The model under review builds one solid part; all positions refer to its coordinate system, in mm. Face numbers are marked on the shaded views. A direction names the side the tool comes from. Round coordinates to 2 decimals unless told otherwise and drop trailing zeros. Order: outer loops, then holes, each group sorted by start corner. A loop starts at its lowest first (then second) coordinate and runs counter-clockwise, first axis right, second up. Notation, with made-up numbers: M -1.75,81 L 47.25,81 A25 ccw 47.25,109 Z; hole C 47,4.5 d9. An arc over 180 degrees is marked long. Answer as a JSON object with one key per item and string values. Group by question number.
1) For the marked faces 4 and 5, list the 3-axis set-ups (+Z, -Z, +X, -X, +Y, -Y) from which the entire face can be reached by the end or side of a thin tool; tool diameter is ignored.
2) To check wall thickness, follow line 1 (Y direction, x = 1.5, z = 3.75); line 2 (X direction, y = 85.5, z = 4); line 3 (X direction, y = 93, z = 8). State the ranges of each line that lie inside material, in increasing order.
3) Consider section A-A, the plane x = -28.5. Write out the cut boundary in (y, z).
4) Insertion check: pin 1 Ø8 at (x, y) = (-24.5, 39.5) entering from +Z; pin 2 Ø2.5 at (x, z) = (-26.5, 6) entering from +Y; pin 3 Ø3 at (y, z) = (50, 4.5) entering from -X; pin 4 Ø2.5 at (x, y) = (-29.5, 117) entering from +Z. Each pin has a flat end and moves straight along its axis. Give the tip position at first contact, or say it passes through.
5) Consider section B-B, the plane y = 38. Write out the cut boundary in (x, z).
6) The part is to be moulded in two halves that separate along Y. For the marked faces 1, 2 and 3, say which applies: +Y half, -Y half, draft (parallel to the pull), parting line (faces both ways), or undercut.
```python
from build123d import *

# Parameters (mm, degrees)
F0_W      = 79.5
F0_H      = 118.5
F1_DEPTH  = 10
F3_R      = 7
F5_DEPTH  = 3.5
F6_R      = 0.8
F8_DEPTH  = 3.5
F9_R      = 2
F10_DEPTH = 4.5
F2_W      = 14.5
F2_H      = 4.5
F11_DEPTH = 4
F13_DEPTH = 9
F14_DEPTH = 25
F15_R     = 2


with BuildPart() as f1:
    # F0 (on Top) → F1 (new body)
    with BuildSketch(Plane.XY):
        with Locations((0, 59.25)):
            Rectangle(F0_W, F0_H)
    extrude(amount=F1_DEPTH)

    # F3
    f3_edges = [f1.edges().sort_by_distance(p)[0] for p in [
        (-39.75, 118.5, 5),
        (-39.75, 0, 5),
        (39.75, 0, 5),
        (39.75, 118.5, 5),
    ]]
    fillet(f3_edges, radius=F3_R)

    # F4 (on face) → F5 (cut)
    with BuildSketch(Plane.XY.offset(10)):
        with BuildLine():
            Line((32.75, 116.5), (-32.75, 116.5))
            ThreePointArc((-32.75, 116.5), (-36.2855339059, 115.0355339059), (-37.75, 111.5))
            Line((-37.75, 111.5), (-37.75, 7))
            ThreePointArc((-37.75, 7), (-36.2855339059, 3.4644660941), (-32.75, 2))
            Line((-32.75, 2), (32.75, 2))
            ThreePointArc((32.75, 2), (36.2855339059, 3.4644660941), (37.75, 7))
            Line((37.75, 7), (37.75, 111.5))
            ThreePointArc((37.75, 111.5), (36.2855339059, 115.0355339059), (32.75, 116.5))
        make_face()
    extrude(amount=-F5_DEPTH, mode=Mode.SUBTRACT)

    # F6
    f6_edges = [f1.edges().sort_by_distance(p)[0] for p in [
        (0, 118.5, 0),
        (37.699747, 116.449747, 0),
        (-37.699747, 116.449747, 0),
        (39.75, 59.25, 0),
        (-39.75, 59.25, 0),
        (37.699747, 2.050253, 0),
        (-37.699747, 2.050253, 0),
        (0, 0, 0),
    ]]
    fillet(f6_edges, radius=F6_R)

    # F7 (on face) → F8 (join)
    with BuildSketch(Plane.XY.offset(6.5)):
        Polygon((-36.25, 100.5), (-37.75, 102), (-37.75, 16.5), (-36.25, 18), align=None)
        Polygon((37.75, 16.5), (37.75, 102), (36.25, 100.5), (36.25, 18), align=None)
        Polygon((-21.75, 3.5), (-23.25, 2), (23.25, 2), (21.75, 3.5), align=None)
        Polygon((23.25, 116.5), (-16.75, 116.5), (-15.25, 115), (21.75, 115), align=None)
    extrude(amount=F8_DEPTH)

    # F9
    f9_edges = [f1.edges().sort_by_distance(p)[0] for p in [
        (-37.75, 102, 8.25),
        (-36.25, 100.5, 8.25),
        (-37.75, 16.5, 8.25),
        (-36.25, 18, 8.25),
        (36.25, 100.5, 8.25),
        (37.75, 102, 8.25),
        (36.25, 18, 8.25),
        (37.75, 16.5, 8.25),
        (23.25, 2, 8.25),
        (21.75, 3.5, 8.25),
        (-23.25, 2, 8.25),
        (-21.75, 3.5, 8.25),
        (-16.75, 116.5, 8.25),
        (-15.25, 115, 8.25),
        (21.75, 115, 8.25),
        (23.25, 116.5, 8.25),
    ]]
    fillet(f9_edges, radius=F9_R)

    # F10 (cut): a face of the model
    f10_faces = [f1.faces().sort_by_distance(p)[0] for p in [
        (-0.0227609258, 59.3168047951, 6.5),
    ]]
    extrude(f10_faces, amount=-F10_DEPTH, mode=Mode.SUBTRACT)

    # F2 (on face) → F11 (cut)
    with BuildSketch(Plane(origin=(0, 118.5, 0), x_dir=(-1, 0, 0), z_dir=(0, 1, 0))):
        with Locations((28.5, 7.75)):
            Rectangle(F2_W, F2_H)
    extrude(amount=-F11_DEPTH, mode=Mode.SUBTRACT)

    # F12 (on face) → F13 (join)
    with BuildSketch(Plane.XY.offset(10)):
        with BuildLine():
            ThreePointArc((-39.75, 92.8803269811), (-40.5, 94.3164676428), (-39.75, 95.7526083044))
            Line((-39.75, 95.7526083044), (-39.75, 101.5))
            Line((-39.75, 101.5), (-41.75, 99.5))
            Line((-41.75, 99.5), (-41.75, 89.7678693718))
            Line((-41.75, 89.7678693718), (-39.75, 87.7678693718))
            Line((-39.75, 87.7678693718), (-39.75, 92.8803269811))
        make_face()
    extrude(amount=-F13_DEPTH)

    # F12 (on face) → F14 (cut)
    with BuildSketch(Plane.XY.offset(10)):
        with BuildLine():
            Line((-39.75, 92.8803269811), (-39.75, 95.7526083044))
            ThreePointArc((-39.75, 95.7526083044), (-40.5, 94.3164676428), (-39.75, 92.8803269811))
        make_face()
        with BuildLine():
            ThreePointArc((-39.75, 92.8803269811), (-37.9399074127, 92.765258437), (-37, 94.3164676428))
            ThreePointArc((-37, 94.3164676428), (-37.9399074127, 95.8676768485), (-39.75, 95.7526083044))
            Line((-39.75, 95.7526083044), (-39.75, 92.8803269811))
        make_face()
    extrude(amount=-F14_DEPTH, mode=Mode.SUBTRACT)

    # F15
    f15_edges = [f1.edges().sort_by_distance(p)[0] for p in [
        (-41.75, 99.5, 5.5),
        (-39.75, 101.5, 5.5),
        (-41.75, 89.767869, 5.5),
        (-39.75, 87.767869, 5.5),
    ]]
    fillet(f15_edges, radius=F15_R)


solid = f1.part
```
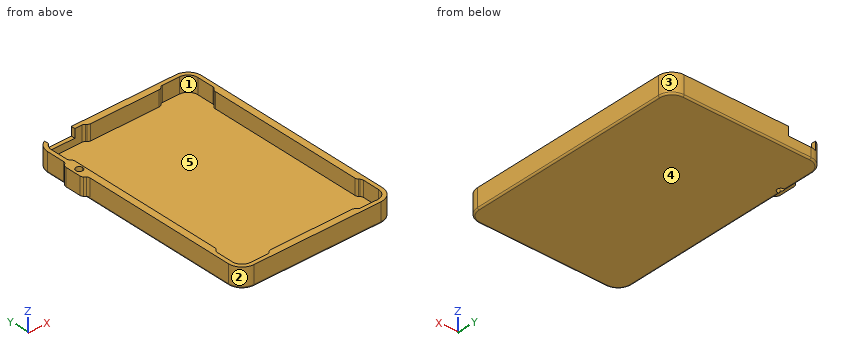
Results list:
{
 "1": {"face 4": "-Z, +X, -X, +Y, -Y", "face 5": "+Z"},
 "2": {"line 1": "0 to 3.5, 115 to 118.5", "line 2": "-39.75 to -36.25, 36.25 to 39.75", "line 3": "-41.75 to -39.9, -37.6 to -36.25, 36.25 to 39.75"},
 "3": {"outline": "M 0,0.8 A0.8 ccw 0.8,0 L 117.7,0 A0.8 ccw 118.5,0.8 L 118.5,5.5 L 116.5,5.5 L 116.5,2 L 2,2 L 2,10 L 0,10 Z"},
 "4": {"pin 1": "z = 2", "pin 2": "y = 118.5", "pin 3": "x = -39.75", "pin 4": "z = 5.5"},
 "5": {"outline": "M -39.75,0.8 A0.8 ccw -38.95,0 L 38.95,0 A0.8 ccw 39.75,0.8 L 39.75,10 L 36.25,10 L 36.25,2 L -36.25,2 L -36.25,10 L -39.75,10 Z"},
 "6": {"face 1": "undercut", "face 2": "-Y half", "face 3": "+Y half"}
}
